Verification items for this drawing (mm, ordinates from the low corner). Round coordinates to 2 decimals unless told otherwise and drop trailing zeros. Order: outer loops, then holes, each group sorted by start corner. A loop starts at its lowest first (then second) coordinate and runs counter-clockwise, first axis right, second up. Notation, with made-up numbers: (-0.5, -33.75) -> (3.5, -33.75) arc R37 ccw to (3.5, 3.25) -> close; hole circle Ø11 at (60.5, 56.25). An arc over 180 degrees is marked (long way). Return JSON: item names as keys, results as strings. Group by question number.
Item 1: Sectioned sample at C-C on z = 0.4. Record the cut outline in (x, y).
Item 2: Scan lines: probe 1 along Y at (x, z) = (5, 0.75); probe 2 along Y at (x, z) = (6.25, 2.1); probe 3 along X at (y, z) = (8.75, 1.6). Record each from-to range of solid material in increasing order. Write a range as from..to.
Item 3: Sectioned sample at A-A on y = 7.5. Record the cut outline in (x, z).
Item 4: Draft check along X on the marked faces 1, 2, 3 and 4. Enter one of: pulls with the +X half, pulls with the -X half, needs draft (parallel to the pull), parting line crosses it, or undercut.
Item 5: Depth check by flat-ended pin: pin 1 Ø3.5 at (x, y) = (5, 7.5) entering from -Z. Enter the tip coordinate at first touch or a pass-through.
Item 6: Sectioned sample at B-B on x = 5. Record the cut outline in (y, z).
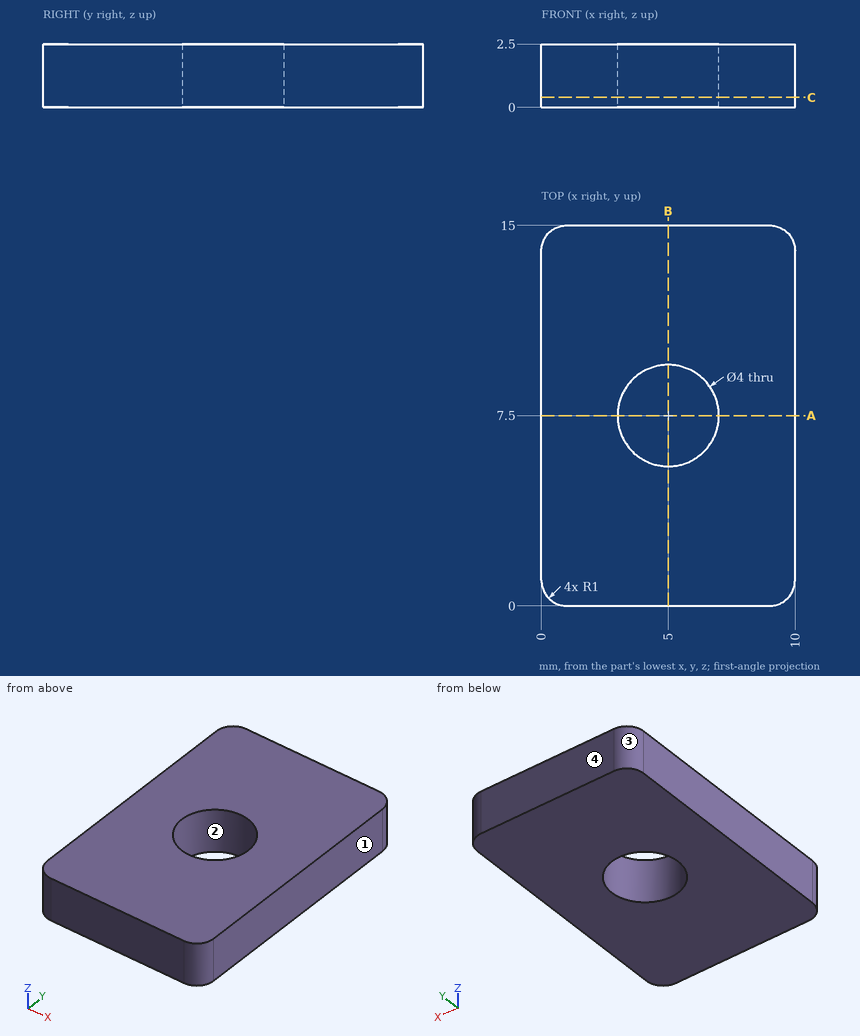
Recorded:
{
 "1": {"outline": "(0, 1) arc R1 ccw to (1, 0) -> (9, 0) arc R1 ccw to (10, 1) -> (10, 14) arc R1 ccw to (9, 15) -> (1, 15) arc R1 ccw to (0, 14) -> close; hole circle Ø4 at (5, 7.5)"},
 "2": {"probe 1": "0..5.5, 9.5..15", "probe 2": "0..5.94, 9.06..15", "probe 3": "0..3.44, 6.56..10"},
 "3": {"outline": "(0, 0) -> (3, 0) -> (3, 2.5) -> (0, 2.5) -> close; (7, 0) -> (10, 0) -> (10, 2.5) -> (7, 2.5) -> close"},
 "4": {"face 1": "pulls with the +X half", "face 2": "undercut", "face 3": "pulls with the -X half", "face 4": "needs draft"},
 "5": {"pin 1": "through"},
 "6": {"outline": "(0, 0) -> (5.5, 0) -> (5.5, 2.5) -> (0, 2.5) -> close; (9.5, 0) -> (15, 0) -> (15, 2.5) -> (9.5, 2.5) -> close"}
}
